Design review of the part built by this model. Coordinates are the model's own, in mm. Coordinates: 2 decimals unless noted, no trailing zeros. Order: outer loops, then holes, each group sorted by start corner. A loop starts at its lowest first (then second) coordinate and runs counter-clockwise, first axis right, second up. Notation, with made-up numbers: M -28,-12 L -10,-12 A19 cw -10,16 Z; hole C -23,55 d8. An arc over 180 degrees is marked long. Answer in a Markdown table with one row per item.
from build123d import *

# Parameters (mm, degrees)
SKICA1_R                 = 35
P_IDAT_VYSUNUT_M1_DEPTH  = 3
ODEBRAT_VYSUNUT_M1_DEPTH = 3
ODEBRAT_VYSUNUT_M3_DEPTH = 3


with BuildPart() as part:
    # Skica1 → Přidat vysunutím1 (new body)
    with BuildSketch(Plane(origin=(0, 0, 0), x_dir=(1, 0, 0), z_dir=(0, 1, 0))):
        with Locations(Location((0, 0, 0), (0, 0, 270))):
            Circle(SKICA1_R)
    extrude(amount=P_IDAT_VYSUNUT_M1_DEPTH)

    # Skica2 → Odebrat vysunutím1 (cut)
    with BuildSketch(Plane(origin=(0, 3, 0), x_dir=(1, 0, 0), z_dir=(0, 1, 0))):
        Polygon((2, 23.916521486), (2, 2), (23.916521486, 2), (23.916521486, -2), (2, -2), (2, -23.916521486), (-2, -23.916521486), (-2, -2), (-23.916521486, -2), (-23.916521486, 2), (-2, 2), (-2, 23.916521486), align=None)
    extrude(amount=-ODEBRAT_VYSUNUT_M1_DEPTH, mode=Mode.SUBTRACT)

    # Skica3 → Odebrat vysunutím3 (cut)
    with BuildSketch(Plane(origin=(0, 3, 0), x_dir=(1, 0, 0), z_dir=(0, 1, 0))):
        Polygon((19.798989873, 26.870057685), (26.870057685, 19.798989873), (24.748737342, 17.67766953), (17.67766953, 24.748737342), align=None)
        Polygon((26.870057685, -19.798989873), (19.798989873, -26.870057685), (17.67766953, -24.748737342), (24.748737342, -17.67766953), align=None)
        Polygon((-19.798989873, -26.870057685), (-26.870057685, -19.798989873), (-24.748737342, -17.67766953), (-17.67766953, -24.748737342), align=None)
        Polygon((-26.870057685, 19.798989873), (-19.798989873, 26.870057685), (-17.67766953, 24.748737342), (-24.748737342, 17.67766953), align=None)
    extrude(amount=-ODEBRAT_VYSUNUT_M3_DEPTH, mode=Mode.SUBTRACT)


solid = part.part
(1) Add section C-C, the plane y = 2.3. Give the number of separate pieces and of enclosed holes in the cut face, and give its area (3 significant figures).
Return value:
| item | result |
|---|---|
| separate pieces | 1 |
| enclosed holes | 5 |
| area | 3,360 mm2 |
(2) For line 1 along Z through (x, y) = (25, 2.95); line 2 along X through (y, z) = (0.55, -21); line 3 along Z through (x, y) = (-1, 0.7), list the stretches that pass through material, from the lowest coordinate up. Write a range as from..to.
Return value:
| item | result |
|---|---|
| line 1 | z = -24.49..-21.67, -17.93..17.93, 21.67..24.49 |
| line 2 | x = -28..-25.67, -21.43..-2, 2..21.43, 25.67..28 |
| line 3 | z = -34.99..-23.92, 23.92..34.99 |
(3) Insertion check: pin 1 Ø0.9 at (y, z) = (2, 10) entering from -X; pin 2 Ø0.9 at (x, y) = (15.5, 1.5) entering from -Z; pin 3 Ø0.9 at (y, z) = (2, -17) entering from +X. Each pin has a flat end and moves straight along its axis. Give the tip position at first contact, or say it passes through.
Return value:
| item | result |
|---|---|
| pin 1 | stops at x = -33.67 |
| pin 2 | stops at z = -31.6 |
| pin 3 | stops at x = 30.84 |
(4) Draft analysis for pull direction Z (two halves, no side actions). For faces 1 (the cylindrical face through (-21, 1, -28)), 2 (the flat face through (-23.917, 2, 0)), 3 (the flat face through (-7, 3, 7)), state which applies: pulls with the +Z half, pulls with the -Z half, needs draft (parallel to the pull), parting line crosses it, or undercut.
Return value:
| item | result |
|---|---|
| face 1 | parting line crosses it |
| face 2 | undercut |
| face 3 | needs draft |
(5) Add section A-A, the plane x = 0. Give the boundary of the cut face in (y, z), and give its area (3 significant figures).
Return value:
| item | result |
|---|---|
| outline | M 0,-35 L 3,-35 L 3,-23.92 L 0,-23.92 Z; M 0,23.92 L 3,23.92 L 3,35 L 0,35 Z |
| area | 66.5 mm2 |
(6) Add section B-B, the plane z = 0. Give the boundary of the cut face in (x, y).
Return value:
| item | result |
|---|---|
| outline | M -35,0 L -23.92,0 L -23.92,3 L -35,3 Z; M 23.92,0 L 35,0 L 35,3 L 23.92,3 Z |
(7) Add section D-D, the plane z = -19. Give the boundary of the cut face in (x, y), and give its area (3 significant figures).
Return value:
| item | result |
|---|---|
| outline | M -29.39,0 L -26.07,0 L -26.07,3 L -29.39,3 Z; M -23.43,0 L -2,0 L -2,3 L -23.43,3 Z; M 2,0 L 23.43,0 L 23.43,3 L 2,3 Z; M 26.07,0 L 29.39,0 L 29.39,3 L 26.07,3 Z |
| area | 148 mm2 |
